from build123d import *

# Parameters (mm, degrees)
SKETCH1_R           = 13
SKETCH1_R_2         = 2
SKETCH1_R_3         = 2.5
BOSS_EXTRUDE1_DEPTH = 9
CUT_EXTRUDE2_START  = -4.3
SKETCH3_R           = 3.25
CUT_EXTRUDE2_DEPTH  = 4.3
FILLET1_R           = 2


with BuildPart() as part:
    # Sketch1 → Boss-Extrude1 (new body)
    with BuildSketch(Plane(origin=(0, 0, 0), x_dir=(1, 0, 0), z_dir=(0, 1, 0))):
        with BuildLine():
            Line((-4.032667043, 28.739999939), (-16.497272732, 15.299999752))
            ThreePointArc((-16.497272732, 15.299999752), (-22.5, 0), (-16.497272732, -15.299999752))
            Line((-16.497272732, -15.299999752), (-4.032667043, -28.739999939))
            ThreePointArc((-4.032667043, -28.739999939), (-3.38e-07, -30.499999725), (4.03266618, -28.740000061))
            Line((4.03266618, -28.740000061), (16.497272272, -15.300000248))
            ThreePointArc((16.497272272, -15.300000248), (22.5, 0), (16.497272272, 15.300000248))
            Line((16.497272272, 15.300000248), (4.03266618, 28.740000061))
            ThreePointArc((4.03266618, 28.740000061), (-4.58e-07, 30.5), (-4.032667043, 28.739999939))
        make_face()
        with Locations(Location((0, 0, 0), (0, 0, 270))):
            Circle(SKETCH1_R, mode=Mode.SUBTRACT)
        with Locations(Location((0, 16, 0), (0, 0, 270))):
            Circle(SKETCH1_R_2, mode=Mode.SUBTRACT)
        with Locations(Location((13.856406461, 8, 0), (0, 0, 270))):
            Circle(SKETCH1_R_2, mode=Mode.SUBTRACT)
        with Locations(Location((13.856406461, -8, 0), (0, 0, 270))):
            Circle(SKETCH1_R_2, mode=Mode.SUBTRACT)
        with Locations(Location((0, -16, 0), (0, 0, 270))):
            Circle(SKETCH1_R_2, mode=Mode.SUBTRACT)
        with Locations(Location((-13.856406461, -8, 0), (0, 0, 270))):
            Circle(SKETCH1_R_2, mode=Mode.SUBTRACT)
        with Locations(Location((-13.856406461, 8, 0), (0, 0, 270))):
            Circle(SKETCH1_R_2, mode=Mode.SUBTRACT)
        with Locations(Location((-3.76e-07, 25, 0), (0, 0, 270))):
            Circle(SKETCH1_R_3, mode=Mode.SUBTRACT)
        with Locations(Location((0, -25, 0), (0, 0, 270))):
            Circle(SKETCH1_R_3, mode=Mode.SUBTRACT)
    extrude(amount=BOSS_EXTRUDE1_DEPTH)

    # Sketch3 → Cut-Extrude2 (cut)
    with BuildSketch(Plane.XZ.offset(CUT_EXTRUDE2_START)):
        with Locations((0, -16)):
            Circle(SKETCH3_R)
        with Locations((-13.856406461, -8)):
            Circle(SKETCH3_R)
        with Locations((-13.856406461, 8)):
            Circle(SKETCH3_R)
        with Locations((0, 16)):
            Circle(SKETCH3_R)
        with Locations((13.856406461, 8)):
            Circle(SKETCH3_R)
        with Locations((13.856406461, -8)):
            Circle(SKETCH3_R)
    extrude(amount=CUT_EXTRUDE2_DEPTH, mode=Mode.SUBTRACT)

    # Fillet1
    fillet1_edges = [part.edges().sort_by_distance(p)[0] for p in [
        (-11.778881987, 2.15, -5.500721691),
        (-10.653205718, 2.15, -7.450450184),
        (-10.653205718, 2.15, 7.450450184),
        (-11.778881987, 2.15, 5.500721691),
        (1.12567627, 2.15, 12.951171875),
        (-1.12567627, 2.15, 12.951171875),
        (11.778881987, 2.15, 5.500721691),
        (10.653205718, 2.15, 7.450450184),
        (10.653205718, 2.15, -7.450450184),
        (11.778881987, 2.15, -5.500721691),
        (-1.12567627, 2.15, -12.951171875),
        (1.12567627, 2.15, -12.951171875),
    ]]
    fillet(fillet1_edges, radius=FILLET1_R)


solid = part.part
Geometry check sheet. Reference: the model listing, model coordinates, mm. A direction names the side the tool comes from. Coordinates: 2 decimals unless noted, no trailing zeros. Order: outer loops, then holes, each group sorted by start corner. A loop starts at its lowest first (then second) coordinate and runs counter-clockwise, first axis right, second up. Notation, with made-up numbers: (27.25, 84) -> (78.25, 84) arc R26 cw to (78.25, 117) -> close; hole circle Ø1 at (77.25, 74). An arc over 180 degrees is marked (long way). Use a Markdown table: item, result. Add a question column.
1. Cross-section at C-C (z = -8). Enter the section's corners in (x, y), and give its area (3 significant figures).
2. Set-up check for faces 5 (the face through (-0.09, 2.18, -19.25)), 6 (the face through (-12.5, 6.62, 6.53)): record each of +Z, -Z, +X, -X, +Y, -Y from which the full face is reachable in a straight line by a thin tool's end or side.
3. Cross-section at A-A (z = 0). Enter the section's corners in (x, y), and give its area (3 significant figures).
4. Mould release check, pull along X, two halves, no side actions. Record for faces 1 (the face through (22.5, 4.4, 0.2)), 2 (the face through (-22.5, 4.4, -0.2)), 3 (the face through (-0.1, 4.4, 30.5)), 4 (the face through (-1.774, 6.617, 16.923)): pulls with the +X half, pulls with the -X half, needs draft (parallel to the pull), parting line crosses it, or undercut.
5. Cross-section at D-D (y = 7.5). Give the number of separate pieces and of enclosed holes in the cut face, and give its area (3 significant figures).
6. Cross-section at B-B (x = 1). Enter the section's corners in (y, z).
7. Material ranges on L1, parallel to Z at x = 2, y = 2; L2, parallel to X at y = 5.45, z = -16; L3, parallel to Z at x = 14.5, y = 5.5, recorded low to high.
8. Go/stop test with flat-tipped pins: pin 1 Ø1.5 at (y, z) = (3, 6.5) entering from -X; pin 2 Ø5 at (x, y) = (17.5, 6) entering from -Z; pin 3 Ø6 at (x, z) = (13.86, 8) entering from -Y; pin 4 Ø10.5 at (x, z) = (-13.86, -8) entering from +Y. Record where each tip stops, or that it passes through.
Filled sheet:
| question | item | result |
|---|---|---|
| 1 | outline | (-21.03, 0) -> (-17.11, 0) -> (-17.11, 4.3) -> (-15.86, 4.3) -> (-15.86, 9) -> (-21.03, 9) -> close; (-11.86, 4.3) -> (-10.25, 4.3) -> (-10.25, 9) -> (-11.86, 9) -> close; (10.25, 4.3) -> (11.86, 4.3) -> (11.86, 9) -> (10.25, 9) -> close; (15.86, 4.3) -> (17.11, 4.3) -> (17.11, 0) -> (21.03, 0) -> (21.03, 9) -> (15.86, 9) -> close |
| 1 | area | 97.5 mm2 |
| 2 | face 5 | -Y |
| 2 | face 6 | +Y, -Y |
| 3 | outline | (-22.5, 0) -> (-13, 0) -> (-13, 9) -> (-22.5, 9) -> close; (13, 0) -> (22.5, 0) -> (22.5, 9) -> (13, 9) -> close |
| 3 | area | 171 mm2 |
| 4 | face 1 | pulls with the +X half |
| 4 | face 2 | pulls with the -X half |
| 4 | face 3 | parting line crosses it |
| 4 | face 4 | undercut |
| 5 | separate pieces | 1 |
| 5 | enclosed holes | 9 |
| 5 | area | 1,190 mm2 |
| 6 | outline | (0, -30.41) -> (9, -30.41) -> (9, -27.29) -> (0, -27.29) -> close; (0, -22.71) -> (9, -22.71) -> (9, -17.73) -> (4.3, -17.73) -> (4.3, -19.09) -> (0, -19.09) -> close; (0, 19.09) -> (4.3, 19.09) -> (4.3, 17.73) -> (9, 17.73) -> (9, 22.71) -> (0, 22.71) -> close; (0, 27.29) -> (9, 27.29) -> (9, 30.41) -> (0, 30.41) -> close; (4.3, -14.27) -> (9, -14.27) -> (9, -12.96) -> (4.3, -12.96) -> close; (4.3, 12.96) -> (9, 12.96) -> (9, 14.27) -> (4.3, 14.27) -> close |
| 7 | L1 | -30.12 to -26.5, -23.5 to -18.56, 18.56 to 23.5, 26.5 to 30.12 |
| 7 | L2 | -15.85 to -2, 2 to 15.85 |
| 7 | L3 | -17.45 to -9.89, -6.11 to 6.11, 9.89 to 17.45 |
| 8 | pin 1 | x = -21.75 |
| 8 | pin 2 | z = -16.91 |
| 8 | pin 3 | y = 4.3 |
| 8 | pin 4 | y = 9 |
